Design review of the part built by this model. Coordinates are the model's own, in mm. A direction names the side the tool comes from. Give positions to 0.01 mm unless a question says otherwise; leave off trailing zeros. Order: outer loops, then holes, each group sorted by start corner. A loop starts at its lowest first (then second) coordinate and runs counter-clockwise, first axis right, second up. Notation, with made-up numbers: (83.25, 42.25) -> (105.25, 42.25) arc R22 cw to (105.25, 70.25) -> close; hole circle Ø1 at (76, 77). An arc over 180 degrees is marked (long way). One line per item, written item: value.
from build123d import *

# Parameters (mm, degrees)
CUT_EXTRUDE1_DEPTH = 5
FILLET1_R          = 1.5


with BuildPart() as part:
    # Sketch1 → Revolve1 (revolve)
    with BuildSketch(Plane.XY, mode=Mode.PRIVATE) as revolve1_sk:
        with BuildLine():
            Line((-1, 35), (0, 35))
            Line((0, 35), (0, 0))
            Line((0, 0), (-3.000286873, 0))
            Line((-3.000286873, 0), (-4.983763516, 0.703110012))
            ThreePointArc((-4.983763516, 0.703110012), (-8.025665426, -1.379057303), (-9.900003631, -4.553241332))
            Line((-9.900003631, -4.553241332), (-11.400003631, -4.553241332))
            ThreePointArc((-11.400003631, -4.553241332), (-9.044878062, -0.365029449), (-5, 2.228558162))
            Line((-5, 2.228558162), (-5, 40))
            Line((-5, 40), (-1, 40))
            Line((-1, 40), (-1, 35))
        make_face()
    revolve(revolve1_sk.sketch.rotate(Axis((0, -4.474343066, 0), (0, 1, 0)), 270), axis=Axis((0, -4.474343066, 0), (0, 1, 0)))

    # Sketch2 → Cut-Extrude1 (cut)
    with BuildSketch(Plane.XZ):
        with BuildLine():
            ThreePointArc((1.5, 2), (0, 2.5), (-1.5, 2))
            Line((-1.5, 2), (1.5, 2))
        make_face()
        Polygon((-1.5, 2), (1.5, 2), (1.5, -2), align=None)
        Polygon((-1.5, 2), (1.5, -2), (-1.5, -2), align=None)
        with BuildLine():
            ThreePointArc((-1.5, -2), (0, -2.5), (1.5, -2))
            Line((1.5, -2), (-1.5, -2))
        make_face()
    extrude(amount=-CUT_EXTRUDE1_DEPTH, mode=Mode.SUBTRACT)

    # Fillet1
    fillet1_edges = [part.edges().sort_by_distance(p)[0] for p in [
        (0, 40, 1),
    ]]
    fillet(fillet1_edges, radius=FILLET1_R)


solid = part.part
Item 1: Add section A-A on y = 4.5. Give the boundary of the cut face in (x, z), plus the area to 3 significant figures.
Returned:
outline: circle Ø10 at (0, 0); hole (-1.5, -2) arc R2.5 ccw to (1.5, -2) -> (1.5, 2) arc R2.5 ccw to (-1.5, 2) -> close
area: 64.5 mm²
Item 2: Draft analysis for pull direction X (two halves, no side actions). For faces 4 (the flat face through (-10.2, -4.553, -0.1)), 5 (the cylindrical face through (4.88, 21.38, 1.08)), 6 (the cylindrical face through (0, 2.5, -2.5)), state which applies: pulls with the +X half, pulls with the -X half, needs draft (parallel to the pull), parting line crosses it, or undercut.
Returned:
face 4: needs draft
face 5: parting line crosses it
face 6: undercut
Item 3: Clearance check with flat-ended pins moving along their axes: P1, Ø1.6, axis at x = 0, z = -0.5, coming from the +Y side; P2, Ø2, axis at y = 3.5, z = 0.5, coming from the -X side; P3, Ø1.5, axis at x = 0.5, z = 0.5, coming from the -Y side. State where each tip first meets the part, or that it passes through.
Returned:
P1: y = 39.4
P2: x = -5
P3: y = 5
Item 4: Add section B-B on y = 32. Give the boundary of the cut face in (x, z), plus the area to 3 significant figures.
Returned:
outline: circle Ø10 at (0, 0)
area: 78.5 mm²
Item 5: Machinability: for faces 1 (the cylindrical face through (0, 2.5, 2.5)), 2 (the cylindrical face through (1, 37, 0)), 3 (the flat face through (2, 40, -2)), which of the approach directions +Z, -Z, +X, -X, +Y, -Y give a long, thin tool a straight path to every point of the face, cutting with its end or side? Answer none if there is none.
Returned:
face 1: -Y
face 2: +Y
face 3: +Z, -Z, +X, -X, +Y
Item 6: To check wall thickness, follow line 1 along X through (y, z) = (35.8, 0); line 2 along Z through (x, y) = (-4, 17); line 3 along X through (y, z) = (-3, 8.25). State the ranges of each line that lie inside material, in increasing order. Write a range as from..to.
Returned:
line 1: -5..-1, 1..5
line 2: -3..3
line 3: -7.02..-4.11, 4.11..7.02
